```python
from build123d import *

# Parameters (mm, degrees)
F0_W      = 38.1
F0_H      = 9.525
F1_DEPTH  = 19.05
F3_D      = 2.2606
F4_W      = 9.525
F4_H      = 9.525
F5_DEPTH  = 9.526
F7_DEPTH  = 19.051
F8_R      = 4.7625
F9_R      = 3.96875
F10_DEPTH = 4.7625


with BuildPart() as f1:
    # F0 (on Top) → F1 (new body)
    with BuildSketch(Plane.XY):
        with Locations((19.05, 4.7625)):
            Rectangle(F0_W, F0_H)
    extrude(amount=F1_DEPTH)

    # F3 (through all)
    with Locations(Plane.XY.offset(19.05)):
        with Locations((15.875, 4.7625), (31.75, 4.7625)):
            Hole(F3_D / 2)

    # F4 (on face) → F5 (cut, through all)
    with BuildSketch(Plane.XZ):
        with Locations((4.7625, 9.525)):
            Rectangle(F4_W, F4_H)
    extrude(amount=-F5_DEPTH, mode=Mode.SUBTRACT)

    # F6 (on face) → F7 (cut, through all)
    with BuildSketch(Plane.XY.offset(19.05)):
        with BuildLine():
            ThreePointArc((2.38125, 4.7625), (4.7625, 2.38125), (7.14375, 4.7625))
            ThreePointArc((7.14375, 4.7625), (4.7625, 7.14375), (2.38125, 4.7625))
        make_face()
    extrude(amount=-F7_DEPTH, mode=Mode.SUBTRACT)

    # F8
    f8_edges = [f1.edges().sort_by_distance(p)[0] for p in [
        (0, 9.525, 16.66875),
        (0, 9.525, 2.38125),
    ]]
    fillet(f8_edges, radius=F8_R)

    # F9 (on face) → F10 (cut)
    with BuildSketch(Plane(origin=(0, 9.525, 0), x_dir=(-1, 0, 0), z_dir=(0, 1, 0))):
        with Locations((-23.8125, 9.525)):
            Circle(F9_R)
    extrude(amount=-F10_DEPTH, mode=Mode.SUBTRACT)


solid = f1.part
```
Input: part model. Units: mm. Frame: model coordinates. A direction names the side the tool comes from. Round coordinates to 2 decimals unless told otherwise and drop trailing zeros. Loops run counter-clockwise (first coordinate to the right, second up) from the corner with the lowest first, then second, coordinate; pieces in that order, holes last. Notation, with made-up numbers: (19.5, 62.25) - (33.5, 62.25) arc R22 cw to (33.5, 89.25) - close; hole circle Ø8 at (49, 60.5). An arc over 180 degrees is marked (long way). One line per item, written item: value. Start each with the question number.
(1) Contact query for flat-ended pins moving along their axis: P1, Ø5, axis at x = 23.81, z = 9.52, coming from the +Y side; P2, Ø1, axis at x = 4.5, y = 3, coming from the -Z side; P3, Ø5, axis at y = 2.5, z = 11, coming from the -X side (3 decimals). Output: stop coordinate, or through.
(2) Access query for faces 1 (the flat face through (9.525, 5, 9)), 2 (the flat face through (24, 4.762, 10)), 3 (the cylindrical face through (4.246, 2.438, 2.415)). Directions: +Z, -Z, +X, -X, +Y, -Y. A direction counts if a zero-diameter tool reaches every point of the face in a straight line with its end or side. Return the directions, or none.
(3) Ray query, line 1 (Y direction, x = 16, z = 16.75) (3 decimals); line 2 (Z direction, x = 8, y = 6.5); line 3 (Y direction, x = 20.5, z = 9.5). Return the intervals inside material, ascending. Write a range as [from, to].
(4) Section C-C, the plane x = 31.75. Return loops of the section in (y, z) (3 decimals).
(5) Draft query along Z for faces 4 (the cylindrical face through (20.15, 7.18, 8)), 5 (the flat face through (19, 5, 19.05)), 6 (the flat face through (38.1, 5, 9)). Return one class per face: +Z half, -Z half, draft (parallel to the pull), parting line (faces both ways), or undercut.
(6) Section B-B, the plane y = 6.75. Count the separate pieces of the cut face and the enclosed holes in it, plus the area to 3 significant figures.
Results below:
1. P1: y = 4.76
1. P2: through
1. P3: x = 9.525
2. face 1: -X, +Y, -Y
2. face 2: +Y
2. face 3: +Z, -Z
3. line 1: [0, 3.639], [5.886, 9.525]
3. line 2: [0, 4.76], [14.29, 19.05]
3. line 3: [0, 4.76]
4. outline: (0, 0) - (3.632, 0) - (3.632, 19.05) - (0, 19.05) - close; (5.893, 0) - (9.525, 0) - (9.525, 19.05) - (5.893, 19.05) - close
5. face 4: undercut
5. face 5: +Z half
5. face 6: draft
6. separate pieces: 3
6. enclosed holes: 1
6. area: 556 mm^2
